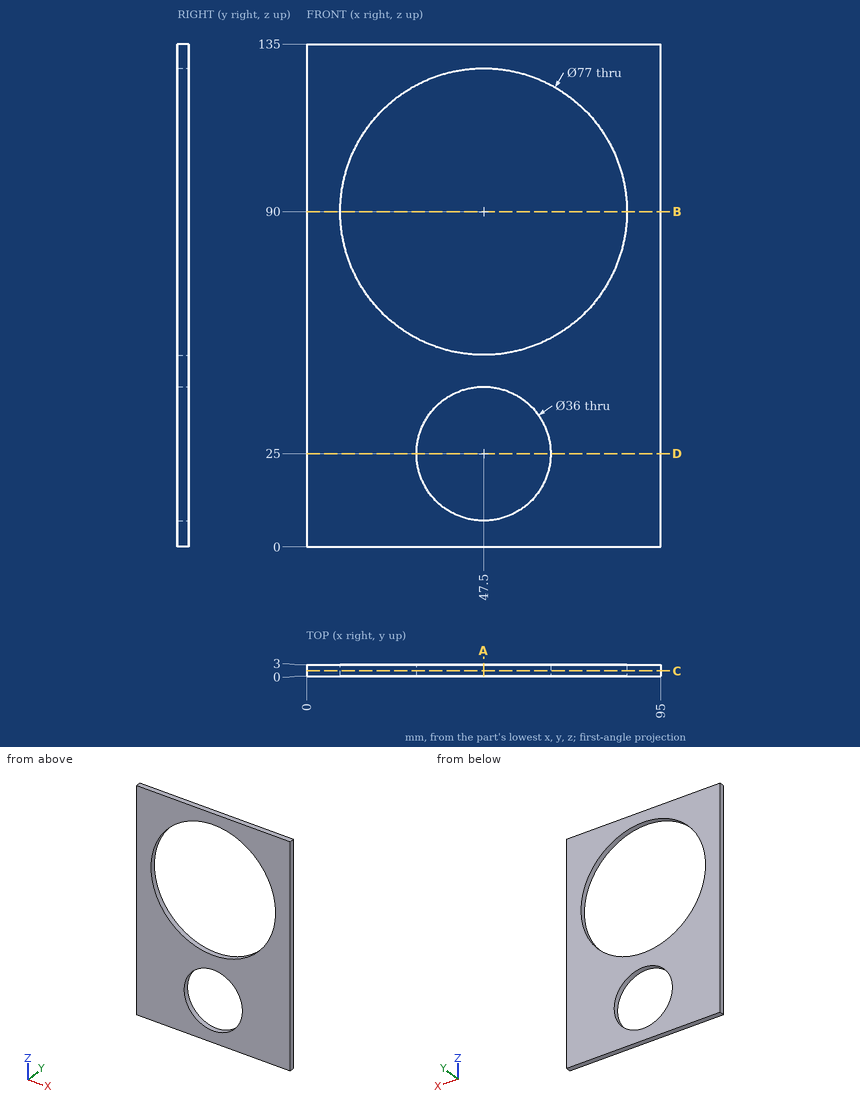
Study the drawing (mm; zero at the part's minimum x, y, z) and answer. Coordinates: 2 decimals unless noted, no trailing zeros. Write each loop counter-clockwise with the first axis right and the second up, starting at its lowest first coordinate (ties: lowest second). Pieces come first, ordered by that corner, then holes. Notation, with made-up numbers: (42, 88) - (86, 88) arc R13 cw to (86, 100) - close; hole circle Ø8 at (85.25, 57.5). An arc over 180 degrees is marked (long way). One line per question, with ' | ' between items.
1) Find section A-A, the plane x = 47.5. Determine the outline of the cut face in (y, z), and give its area (3 significant figures).
Checks:
outline: (0, 0) - (3, 0) - (3, 7) - (0, 7) - close; (0, 43) - (3, 43) - (3, 51.5) - (0, 51.5) - close; (0, 128.5) - (3, 128.5) - (3, 135) - (0, 135) - close | area: 66.0 mm2
2) Find section B-B, the plane z = 90. Determine the outline of the cut face in (x, y).
Checks:
outline: (0, 0) - (9, 0) - (9, 3) - (0, 3) - close; (86, 0) - (95, 0) - (95, 3) - (86, 3) - close
3) Find section C-C, the plane y = 1.4. Determine the outline of the cut face in (x, z), and give its area (3 significant figures).
Checks:
outline: (0, 0) - (95, 0) - (95, 135) - (0, 135) - close; hole circle Ø77 at (47.5, 90); hole circle Ø36 at (47.5, 25) | area: 7,150 mm2
4) Find section D-D, the plane z = 25. Determine the outline of the cut face in (x, y), and give its area (3 significant figures).
Checks:
outline: (0, 0) - (29.5, 0) - (29.5, 3) - (0, 3) - close; (65.5, 0) - (95, 0) - (95, 3) - (65.5, 3) - close | area: 177 mm2
5) A flat-ended cylindrical pin translates along its axis: P1, Ø1, axis at y = 0.5, z = 120.5, coming from the -X side. Find the tip coordinate at first contact, or state that the pin passes through.
Checks:
P1: x = 0
6) Consider probe 1 along Z at (x, y) = (47.5, 0.95); probe 2 along X at (y, z) = (1.5, 25); probe 3 along X at (y, z) = (1.7, 90). Determine where each line is inside the solid, lowest interval first. Write a range as [from, to].
Checks:
probe 1: [0, 7], [43, 51.5], [128.5, 135] | probe 2: [0, 29.5], [65.5, 95] | probe 3: [0, 9], [86, 95]
